The listing builds one solid part. Answer for the finished solid, in the listing's coordinates (mm). Face numbers are marked on the shaded views. A direction names the side the tool comes from. Coordinates: 2 decimals unless noted, no trailing zeros. Order: outer loops, then holes, each group sorted by start corner. A loop starts at its lowest first (then second) coordinate and runs counter-clockwise, first axis right, second up. Notation, with made-up numbers: (89.25, 26.25) -> (129.25, 26.25) arc R18 ccw to (129.25, 47.25) -> close; hole circle Ø9 at (-21, 44.25). An arc over 180 degrees is marked (long way). One line per question, with ' | ' between items.
Autodesk Inventor part; units mm, degrees
ref_plane "YZ Plane" through (0, 0, 0) normal (1, 0, 0) x (0, 1, 0)
ref_plane "XZ Plane" through (0, 0, 0) normal (0, 1, 0) x (-1, 0, 0)
ref_plane "XY Plane" through (0, 0, 0) normal (0, 0, 1) x (1, 0, 0)
sketch "Sketch1" plane through (0, 0, 0) normal (0, 0, 1) x (1, 0, 0)
  line L0 (0, 0.1624) -> (0, 12.1749)
  line L1 (0, 12.1749) -> (1.524, 12.1749)
  line L2 (1.524, 12.1749) -> (1.524, 101.0749)
  line L3 (1.524, 101.0749) -> (0, 101.0749)
  line L4 (0, 101.0749) -> (0, 12.1749)
  line L5 (0, 101.0749) -> (1.9875, 101.0749)
  line L6 (1.9875, 101.0749) -> (1.9875, 110.2189)
  line L7 (1.9875, 110.2189) -> (0, 110.2189)
  line L8 (0, 110.2189) -> (0, 101.0749)
  line L9 (0, 110.2189) -> (2.54, 110.2189)
  line L10 (2.54, 110.2189) -> (2.54, 111.4889)
  line L11 (2.54, 111.4889) -> (0, 111.4889)
  line L12 (0, 111.4889) -> (0, 110.2189)
  line L13 (2.54, 111.4889) -> (1.27, 116.5689)
  line L14 (0, 116.5689) -> (0, 111.4889)
  line L15 (0, 116.5689) -> (1.27, 116.5689)
  line L16 (1.143, 116.5689) -> (0.6099, 119.3321)
  line L17 (0, 119.7439) -> (0, 116.5689)
  line L18 (0, 119.7439) -> (0.1111, 119.7439)
  arc A0 (0.6099, 119.3321) -> (0.1111, 119.7439) centre (0.1111, 119.2359) ccw
  point P0 (0, 0)
  point P1 (0.5305, 119.7439)
  dimension "d0" = 1.524
  dimension "d1" = 88.9
  dimension "d2" = 1.9875
  dimension "d3" = 9.144
  dimension "d4" = 2.54
  dimension "d5" = 1.27
  dimension "d6" = 5.08
  dimension "d7" = 1.27
  dimension "d8" = 1.143
  dimension "d9" = 3.175
  dimension "d10" = 0.508
revolve "Revolution1" add sketch "Sketch1" angle 360 about axis through (0, 119.7439, 0) along (0, -1, 0)
properties part number "Ink Barrel + Tip"
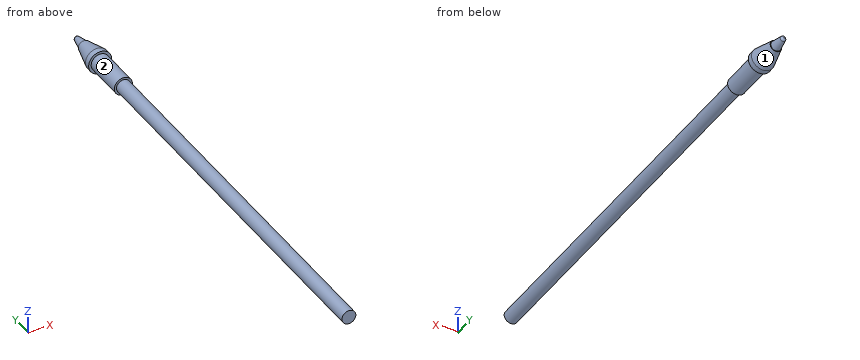
Item 1: Section A-A, the plane y = 52.5 is taken. Give the vertices of the cut face in (x, z), plus the area to 3 significant figures.
Computed values:
outline: circle Ø3.05 at (0, 0) | area: 7.30 mm^2
Item 2: For the marked faces 1 and 2, determine the directions among +Z, -Z, +X, -X, +Y, -Y from which every point of the face is accessible in a straight line to the end or side of a thin tool.
Computed values:
face 1: +Y | face 2: -Y
Item 3: Find the intervals of material crossed by L1, parallel to X at y = 104.5, z = 0.2; L2, parallel to X at y = 100, z = -0.05; L3, parallel to Z at x = 0.35, y = 90, in increasing order.
Computed values:
L1: x = -1.98 to 1.98 | L2: x = -1.52 to 1.52 | L3: z = -1.48 to 1.48
Item 4: Each of these flat-tipped pins is pushed along its axis until it touches: pin 1 Ø3 at (y, z) = (28.5, -2) entering from +X; pin 2 Ø2 at (y, z) = (38, 2) entering from +X; pin 3 Ø1.5 at (x, y) = (0, 64.5) entering from +Z. Where does it stop, or does it pass through?
Computed values:
pin 1: stops at x = 1.44 | pin 2: stops at x = 1.15 | pin 3: stops at z = 1.52
